```python
from build123d import *

# Parameters (mm, degrees)
SKETCH_R        = 7
SKETCH_R_2      = 3.5
PAD_DEPTH       = 25
SKETCH001_R     = 25
PAD001_DEPTH    = 10
SKETCH002_W     = 35
SKETCH002_H     = 36
POCKET_DEPTH    = 30.001
SKETCH003_R     = 7
POCKET001_DEPTH = 25.001
SKETCH004_R     = 6.5
POCKET002_DEPTH = 10.001
SKETCH005_W     = 10
SKETCH005_H     = 50
PAD002_DEPTH    = 10
SKETCH006_R     = 10
POCKET003_DEPTH = 10
SKETCH007_W     = 3
SKETCH007_H     = 30
POCKET004_DEPTH = 80.001


with BuildPart() as part:
    # Sketch → Pad (new body, symmetric)
    with BuildSketch(Plane.XZ):
        with BuildLine():
            Line((0, 0), (0, 5))
            Line((0, 5), (6, 5))
            Line((6, 5), (6, 33))
            ThreePointArc((30, 45), (8.291796, 58.416408), (6, 33))
            Line((30, 10), (30, 45))
            Line((55, 10), (30, 10))
            Line((55, 0), (55, 10))
            Line((0, 0), (55, 0))
        make_face()
        with Locations((15, 45)):
            Circle(SKETCH_R, mode=Mode.SUBTRACT)
        with Locations((18, 10)):
            Circle(SKETCH_R_2, mode=Mode.SUBTRACT)
    extrude(amount=PAD_DEPTH, both=True)

    # Sketch001 (on Face6 of Pad) → Pad001 (join)
    with BuildSketch(Plane(origin=(0, 0, 10), x_dir=(-1, 0, 0), z_dir=(0, 0, 1))):
        with Locations((-55, 0)):
            Circle(SKETCH001_R)
    extrude(amount=-PAD001_DEPTH)

    # Sketch002 (on Face7 of Pad001) → Pocket (cut, through all)
    with BuildSketch(Plane(origin=(30, 0, 0), x_dir=(0, 0, 1), z_dir=(1, 0, 0))):
        with Locations((42.5, 0)):
            Rectangle(SKETCH002_W, SKETCH002_H)
    extrude(amount=-POCKET_DEPTH, mode=Mode.SUBTRACT)

    # Sketch003 (on Face16 of Pocket) → Pocket001 (cut, through all)
    with BuildSketch(Plane(origin=(0, 0, 25), x_dir=(-1, 0, 0), z_dir=(0, 0, 1))):
        with Locations((-17, 0)):
            Circle(SKETCH003_R)
    extrude(amount=-POCKET001_DEPTH, mode=Mode.SUBTRACT)

    # Sketch004 (on Face11 of Pocket001) → Pocket002 (cut, through all)
    with BuildSketch(Plane(origin=(0, 0, 10), x_dir=(-1, 0, 0), z_dir=(0, 0, 1))):
        with Locations((-55, 0)):
            Circle(SKETCH004_R)
    extrude(amount=-POCKET002_DEPTH, mode=Mode.SUBTRACT)

    # Sketch005 (on Face11 of Pocket002) → Pad002 (join)
    with BuildSketch(Plane(origin=(30, 0, 0), x_dir=(0, 0, 1), z_dir=(1, 0, 0))):
        with Locations((15, 0)):
            Rectangle(SKETCH005_W, SKETCH005_H)
    extrude(amount=PAD002_DEPTH)

    # Sketch006 (on Face20 of Pad002) → Pocket003 (cut)
    with BuildSketch(Plane(origin=(40, 0, 0), x_dir=(0, 0, 1), z_dir=(1, 0, 0))):
        with Locations((20, 0)):
            Circle(SKETCH006_R)
    extrude(amount=-POCKET003_DEPTH, mode=Mode.SUBTRACT)

    # Sketch007 (on Face1 of Pocket003) → Pocket004 (cut, through all)
    with BuildSketch(Plane(origin=(0, 0, 0), x_dir=(0, 0, -1), z_dir=(-1, 0, 0))):
        with Locations((-1.5, 0)):
            Rectangle(SKETCH007_W, SKETCH007_H)
    extrude(amount=-POCKET004_DEPTH, mode=Mode.SUBTRACT)


solid = part.part
```
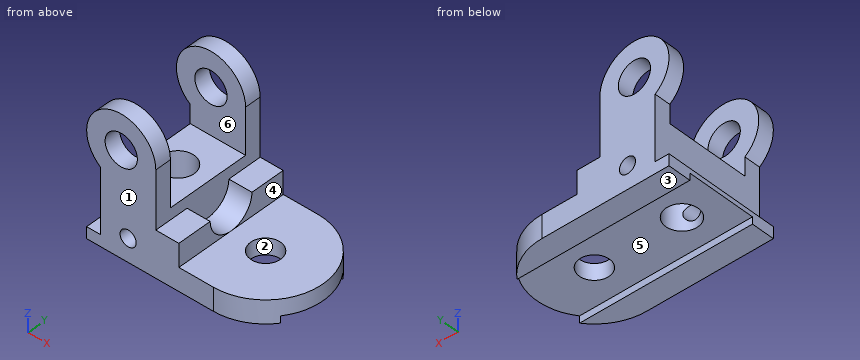
Could you check a few things on this model? Use its own coordinates, in mm. Face numbers are marked on the shaded views. A direction names the side the tool comes from. Give positions to 0.01 mm unless a question says otherwise; leave off trailing zeros. Loops run counter-clockwise (first coordinate to the right, second up) from the corner with the lowest first, then second, coordinate; pieces in that order, holes last. Notation, with made-up numbers: (38.25, 32.5) - (95.25, 32.5) arc R15 ccw to (95.25, 49.5) - close; hole circle Ø11 at (46.5, 3). An arc over 180 degrees is marked (long way). Use one line per item in the form item = value.
1. I want a section at D-D (y = -16.5). Please give me the cut outline in (x, z).
Response values:
outline = (0, 0) - (73.78, 0) - (73.78, 10) - (40, 10) - (40, 20) - (30, 20) - (30, 25) - (6, 25) - (6, 5) - (0, 5) - close; hole circle Ø7 at (18, 10)
2. Thinking about a two-plate mould opening in Y: for the marked faces 1, 2 and 3, which applies, released by +Y, released by -Y, zero draft, split by the parting line, or undercut?
Response values:
face_1 = released by -Y
face_2 = undercut
face_3 = zero draft
3. I'm going to push flat-ended pins straight in: pin 1 Ø4 at (x, y) = (43.5, -4.5) entering from +Z; pin 2 Ø10 at (x, y) = (38.5, 16) entering from +Z; pin 3 Ø5 at (y, z) = (0, 13) entering from +X; pin 4 Ø8 at (y, z) = (7, 30.5) entering from +X. Where does each tip first touch, or does it pass through?
Response values:
pin_1 = 10
pin_2 = 20
pin_3 = 30
pin_4 = through
4. On a 3-axis mill with a long thin cutter (end or side, diameter ignored), from which of +Z, -Z, +X, -X, +Y, -Y can I reach the whole of each face in a straight line? I mean the marked faces 4, 5 and 6. Say none if no direction works.
Response values:
face_4 = +Z, +X, +Y, -Y
face_5 = -Z, +X, -X
face_6 = +Z, +X, -X
5. I want a section at B-B (z = 7.5). Please give me the cut outline in (x, y).
Response values:
outline = (6, -25) - (15.55, -25) - (15.55, -6.85) arc R7 cw to (15.55, 6.85) - (15.55, 25) - (6, 25) - close; (20.45, -25) - (55, -25) arc R25 ccw to (55, 25) - (20.45, 25) - (20.45, 6.09) arc R7 cw to (20.45, -6.09) - close; hole circle Ø13 at (55, 0)
6. I want a section at C-C (x = 41). Please give me the cut outline in (y, z), and give its area (3 significant figures).
Response values:
outline = (-25, 0) - (-15, 0) - (-15, 3) - (15, 3) - (15, 0) - (25, 0) - (25, 10) - (-25, 10) - close
area = 410 mm²
7. I want a section at A-A (z = 32). Please give me the cut outline in (x, y).
Response values:
outline = (6, -25) - (30, -25) - (30, -18) - (6, -18) - close; (6, 18) - (30, 18) - (30, 25) - (6, 25) - close
8. I need wall thicknesses on probe 1 along X at (y, z) = (21.5, 45); probe 2 along Z at (x, y) = (18, -11.25); probe 3 along Y at (x, z) = (29.5, 40.5). Which ranges of each line are inside material? Lowest first, please.
Response values:
probe_1 = 0 to 8, 22 to 30
probe_2 = 3 to 6.5, 13.5 to 25
probe_3 = -25 to -18, 18 to 25
